Can you work these out from the model? Positions are in its coordinate system, mm. Face numbers are marked on the shaded views. A direction names the side the tool comes from. Round coordinates to 2 decimals unless told otherwise and drop trailing zeros. Order: outer loops, then holes, each group sorted by start corner. A loop starts at its lowest first (then second) coordinate and runs counter-clockwise, first axis right, second up. Notation, with made-up numbers: (-29.5, -36) -> (14.5, -36) arc R20 cw to (14.5, -5) -> close; hole circle Ø2 at (39.5, -22). An arc over 180 degrees is marked (long way). Use a Markdown table: item, result. Add a question column.
Q1. If we section it at A-A on x = 0: List the corners of the cut face in (y, z) for me.
Q2. I'm going to push flat-ended pins straight in: pin 1 Ø14 at (x, z) = (-5, 18.5) entering from -Y; pin 2 Ø8 at (x, z) = (18, 45.5) entering from -Y; pin 3 Ø12 at (x, z) = (16, 58) entering from +Y; pin 4 Ø10 at (y, z) = (-2, 79) entering from +X. Where does each tip first touch, or does it pass through?
Q3. If we section it at B-B on x = -20: List the corners of the cut face in (y, z) for me, plus the area to 3 significant figures.
Q4. We'd pull the mould along Z, two halves only. Please class the marked faces 4, 5 and 6: +Z half, -Z half, draft (parallel to the pull), parting line (faces both ways), or undercut.
Q5. If we section it at D-D on y = 6: List the corners of the cut face in (x, z) for me.
Q6. For the marked faces 1, 2 and 3, which set-ups out of +Z, -Z, +X, -X, +Y, -Y let a thin tool reach every point of the face, with its end or its side?
Q7. I need wall thicknesses on line 1 along X through (y, z) = (8, 0); line 2 along Z through (x, y) = (9, -12.5); line 3 along Z through (x, y) = (10, -17). Which ranges of each line are inside material? Lowest first, please. Write a range as [from, to].
Q8. If we section it at C-C on z = 42: List the corners of the cut face in (x, y) for me, plus the area to 3 significant figures.
Autodesk Inventor part; units mm, degrees
ref_plane "YZ Plane" through (0, 0, 0) normal (1, 0, 0) x (0, 1, 0)
ref_plane "XZ Plane" through (0, 0, 0) normal (0, 1, 0) x (-1, 0, 0)
ref_plane "XY Plane" through (0, 0, 0) normal (0, 0, 1) x (1, 0, 0)
sketch "Boceto1" plane through (0, 0, 0) normal (1, 0, 0) x (0, 1, 0)
  line L0 (-17.5, -25) -> (17.5, -25)
  line L1 (17.5, -25) -> (17.5, 25)
  line L2 (17.5, 25) -> (-17.5, 25)
  line L3 (-17.5, 25) -> (-17.5, -25)
  line L4 (7.5, 25) -> (7.5, 50)
  line L5 (-7.5, 45.9808) -> (-7.5, 25)
  line L6 (17.5, 12.5) -> (-17.5, 12.5)
  line L7 (17.5, -12.5) -> (-17.5, -12.5)
  line L8 (7.5, 50) -> (-17.5, 93.3013)
  line L9 (-17.5, 93.3013) -> (-30.4904, 85.8013)
  line L10 (-30.4904, 85.8013) -> (-7.5, 45.9808)
  line L11 (-40.0885, 0) -> (27.0981, 0)
  point P0 (0, 0)
  dimension "d0" = 10
  dimension "d1" = 10
  dimension "d2" = 15
  dimension "d3" = 25
  dimension "d5" = 12.5
  dimension "d6" = 50
  dimension "d7" = 12.5
  dimension "d8" = 7.5
  dimension "d9" = 25
  dimension "d10" = 50
  dimension "d11" = 15
  dimension "d12" = 150
revolve "Revolución1" add sketch "Boceto1" angle 360 about axis through (0, -10, 0) along (0, 1, 0) contours L3 L2 L1 L6
extrude "Extrusión1" add sketch "Boceto1" along normal mid plane 50 contours L5 L10 L9 L8 L4 L2
sketch "Boceto2" plane through (25, 7.5, 25) normal (0, 0, -1) x (-1, 0, 0)
  line L0 (25, -15) -> (25, 0)
  line L1 (25, 0) -> (0, 0)
  line L2 (0, -15) -> (0, 0)
  line L3 (25, -15) -> (0, -15)
  line L4 (50, -15) -> (25, -15)
  line L5 (50, 0) -> (50, -15)
  line L6 (50, 0) -> (25, 0)
  point P0 (25, -7.5)
extrude "Extrusión2" add sketch "Boceto2" along normal up to surface
sketch "Boceto3" plane through (-25, -17.5, 93.3013) normal (0, 0.866, 0.5) x (1, 0, 0)
  line L0 (0, 0) -> (0, 50)
  line L1 (0, 30) -> (50, 30)
  line L2 (50, 30) -> (50, 20)
  line L3 (50, 0) -> (50, 45.9808)
  line L4 (0, 30) -> (0, 20)
  line L5 (50, 20) -> (0, 20)
  line L6 (0, 50) -> (50, 50)
  circle A0 centre (25, 10) radius 5
  point P0 (25, 89.5513)
  point P1 (0, 25)
  dimension "d18" = 10
  dimension "d19" = 5
  dimension "d20" = 25
  dimension "d21" = 10
  dimension "d22" = 10
extrude "Extrusión3" cut sketch "Boceto3" against normal blind 5 contours L0 L1 L2 L5
extrude "Extrusión4" cut sketch "Boceto3" against normal through all contours A0
properties part number "Pieza de practica 14"
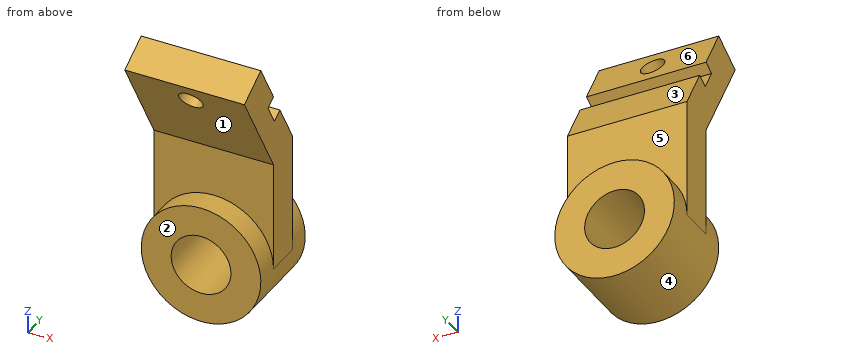
Answer below:
| question | item | result |
|---|---|---|
| 1 | outline | (-30.49, 85.8) -> (-27.99, 81.47) -> (-15, 88.97) -> (-17.5, 93.3) -> close; (-22.99, 72.81) -> (-7.5, 45.98) -> (-7.5, 25) -> (-17.5, 25) -> (-17.5, 12.5) -> (17.5, 12.5) -> (17.5, 25) -> (7.5, 25) -> (7.5, 50) -> (-2.5, 67.32) -> (-6.83, 64.82) -> (-11.83, 73.48) -> (-7.5, 75.98) -> (-10, 80.31) -> close; (-17.5, -25) -> (17.5, -25) -> (17.5, -12.5) -> (-17.5, -12.5) -> close |
| 2 | pin 1 | y = -17.5 |
| 2 | pin 2 | y = -9.53 |
| 2 | pin 3 | y = 6.35 |
| 2 | pin 4 | through |
| 3 | outline | (-30.49, 85.8) -> (-7.5, 45.98) -> (-7.5, 15) -> (-17.5, 15) -> (-17.5, -15) -> (17.5, -15) -> (17.5, 15) -> (7.5, 15) -> (7.5, 50) -> (-2.5, 67.32) -> (-6.83, 64.82) -> (-11.83, 73.48) -> (-7.5, 75.98) -> (-17.5, 93.3) -> close |
| 3 | area | 2,210 mm² |
| 4 | face 4 | undercut |
| 4 | face 5 | draft |
| 4 | face 6 | +Z half |
| 5 | outline | (-25, 0) arc R25 ccw to (25, 0) -> (25, 52.6) -> (-25, 52.6) -> close; hole circle Ø25 at (0, 0) |
| 6 | face 1 | +X, -X, -Y |
| 6 | face 2 | -Z, +X, -X, -Y |
| 6 | face 3 | +Z, +X, -X, +Y |
| 7 | line 1 | [-25, -12.5], [12.5, 25] |
| 7 | line 2 | [-23.32, -8.67], [8.67, 23.32], [54.64, 84.64] |
| 7 | line 3 | [-22.91, -7.5], [7.5, 22.91], [62.44, 92.44] |
| 8 | outline | (-25, -7.5) -> (25, -7.5) -> (25, 7.5) -> (-25, 7.5) -> close |
| 8 | area | 750 mm² |
